Input: part model. Units: mm. Frame: model coordinates. Give positions to 0.01 mm unless a question says otherwise; leave off trailing zeros. Loops run counter-clockwise (first coordinate to the right, second up) from the corner with the lowest first, then second, coordinate; pieces in that order, holes last. Notation, with made-up numbers: (68.25, -18) - (93.25, -18) arc R16 cw to (93.25, -6) - close; hole circle Ø4 at (56, 24). An arc over 180 degrees is marked (long way). Answer as a JSON object with one key per item and string values. Group by question number.
(1) Material intervals for L1, parallel to X at y = 31.5, z = 2.95; L2, parallel to Y at x = -8.5, z = 2.55; L3, parallel to X at y = 29, z = 3.55, sorted ascending.
(2) Mould query, pull axis Y, two halves, no side actions, for faces 1 (the cylindrical face through (9.457, 29.212, 1.972)), 2 (the cylindrical face through (-8.351, 47.095, 1.972)), 3 (the cylindrical face through (-6.11, 49.35, 1.97)). Classes: +Y half, -Y half, draft (parallel to the pull), parting line (faces both ways), or undercut.
(3) Section query C-C (y = 46). Return loops of the section in (x, z).
(4) Pin query (flat end, axial travel): P1, Ø1.5, axis at y = 27.5, z = 1, coming from the +X side; P2, Ø2, axis at x = -2.5, z = 2, coming from the +Y side. Return the tip coordinate at first contact, or that it passes through.
(5) Section query A-A (z = 2.15). Return loops of the section in (x, y), plus the area to 3 significant figures.
(6) Section query B-B (x = 4). Return loops of the section in (y, z), plus the area to 3 significant figures.
```python
from build123d import *

# Parameters (mm, degrees)
BOSS_EXTRUDE1_DEPTH = 4


with BuildPart() as part:
    # Sketch1 → Boss-Extrude1 (new body)
    with BuildSketch(Plane.XY):
        with BuildLine():
            ThreePointArc((-9.405096609, 49.466499285), (-10.662900345, 49.351582329), (-11.909548916, 49.148743758))
            Line((-11.909548916, 49.148743758), (-12.670152398, 46.498155867))
            ThreePointArc((-12.670152398, 46.498155867), (-19.428156186, 42.525600365), (-23.400711687, 35.767596578))
            Line((-23.400711687, 35.767596578), (-26.051299579, 35.006993096))
            ThreePointArc((-26.051299579, 35.006993096), (-26.25413815, 33.760344525), (-26.369055105, 32.502540789))
            ThreePointArc((-26.369055105, 32.502540789), (-24.849782677, 32.78323576), (-23.997290399, 31.494734579))
            ThreePointArc((-23.997290399, 31.494734579), (-24.849782677, 30.206233398), (-26.369055105, 30.486928369))
            ThreePointArc((-26.369055105, 30.486928369), (-26.25413815, 29.229124633), (-26.051299579, 27.982476062))
            Line((-26.051299579, 27.982476062), (-23.400711687, 27.22187258))
            ThreePointArc((-23.400711687, 27.22187258), (-19.428156186, 20.463868792), (-12.670152398, 16.491313291))
            Line((-12.670152398, 16.491313291), (-11.909548916, 13.840725399))
            ThreePointArc((-11.909548916, 13.840725399), (-10.662900345, 13.637886829), (-9.405096609, 13.522969873))
            ThreePointArc((-9.405096609, 13.522969873), (-8.921251899, 15.792988925), (-6.997290399, 14.494734579))
            ThreePointArc((-6.997290399, 14.494734579), (-7.099036053, 13.970773079), (-7.38948419, 13.522969873))
            ThreePointArc((-7.38948419, 13.522969873), (-6.131680454, 13.637886829), (-4.885031883, 13.840725399))
            Line((-4.885031883, 13.840725399), (-4.124428401, 16.491313291))
            ThreePointArc((-4.124428401, 16.491313291), (2.633575387, 20.463868792), (6.606130888, 27.22187258))
            Line((6.606130888, 27.22187258), (9.25671878, 27.982476062))
            ThreePointArc((9.25671878, 27.982476062), (9.459557351, 29.229124633), (9.574474306, 30.486928369))
            ThreePointArc((9.574474306, 30.486928369), (7.202709601, 31.494734579), (9.574474306, 32.502540789))
            ThreePointArc((9.574474306, 32.502540789), (9.459557351, 33.760344525), (9.25671878, 35.006993096))
            Line((9.25671878, 35.006993096), (6.606130888, 35.767596578))
            ThreePointArc((6.606130888, 35.767596578), (2.633575387, 42.525600365), (-4.124428401, 46.498155867))
            Line((-4.124428401, 46.498155867), (-4.885031883, 49.148743758))
            ThreePointArc((-4.885031883, 49.148743758), (-6.131680454, 49.351582329), (-7.38948419, 49.466499285))
            ThreePointArc((-7.38948419, 49.466499285), (-8.397290399, 47.094734579), (-9.405096609, 49.466499285))
        make_face()
    extrude(amount=BOSS_EXTRUDE1_DEPTH)


solid = part.part
```
Recorded:
{
 "1": {"L1": "x = -24 to 7.2", "L2": "y = 15.89 to 47.1", "L3": "x = -26.22 to 9.43"},
 "2": {"face 1": "-Y half", "face 2": "undercut", "face 3": "+Y half"},
 "3": {"outline": "(-14.14, 0) - (-2.66, 0) - (-2.66, 4) - (-14.14, 4) - close"},
 "4": {"P1": "stops at x = 9.31", "P2": "stops at y = 46.31"},
 "5": {"outline": "(-26.37, 30.49) arc R18 ccw to (-26.05, 27.98) - (-23.4, 27.22) arc R15.6 ccw to (-12.67, 16.49) - (-11.91, 13.84) arc R18 ccw to (-9.41, 13.52) arc R1.4 cw (long way) to (-7.39, 13.52) arc R18 ccw to (-4.89, 13.84) - (-4.12, 16.49) arc R15.6 ccw to (6.61, 27.22) - (9.26, 27.98) arc R18 ccw to (9.57, 30.49) arc R1.4 cw (long way) to (9.57, 32.5) arc R18 ccw to (9.26, 35.01) - (6.61, 35.77) arc R15.6 ccw to (-4.12, 46.5) - (-4.89, 49.15) arc R18 ccw to (-7.39, 49.47) arc R1.4 cw (long way) to (-9.41, 49.47) arc R18 ccw to (-11.91, 49.15) - (-12.67, 46.5) arc R15.6 ccw to (-23.4, 35.77) - (-26.05, 35.01) arc R18 ccw to (-26.37, 32.5) arc R1.4 cw (long way) to start", "area": "818 mm^2"},
 "6": {"outline": "(22.03, 0) - (40.96, 0) - (40.96, 4) - (22.03, 4) - close", "area": "75.8 mm^2"}
}
